from build123d import *

# Parameters (mm, degrees)
STOCK_TO_SIZE_DEPTH = 3.175
SKETCH2_R           = 2.286
MOUNTING_HOLE_DEPTH = 4.175


with BuildPart() as part:
    # Sketch1 → Stock to Size (new body)
    with BuildSketch(Plane(origin=(0, 0, 0), x_dir=(1, 0, 0), z_dir=(0, 1, 0))):
        with BuildLine():
            Line((-72.207668016, -239.550243772), (113.425121886, -239.550243772))
            ThreePointArc((113.425121886, -239.550243772), (117.915249947, -237.690371833), (119.775121886, -233.200243772))
            Line((119.775121886, -233.200243772), (119.775121886, 363.699756228))
            ThreePointArc((119.775121886, 363.699756228), (117.915249947, 368.189884288), (113.425121886, 370.049756228))
            Line((113.425121886, 370.049756228), (-154.880183722, 370.049756228))
            Line((-154.880183722, 370.049756228), (-180.160298169, 342.461352424))
            Line((-180.160298169, 342.461352424), (-78.461197248, -234.302909701))
            ThreePointArc((-78.461197248, -234.302909701), (-76.289369337, -238.064625986), (-72.207668016, -239.550243772))
        make_face()
    extrude(amount=STOCK_TO_SIZE_DEPTH)

    # Sketch2 → Mounting Hole (cut, through all)
    with BuildSketch(Plane(origin=(0, 3.175, 0), x_dir=(1, 0, 0), z_dir=(0, 1, 0))):
        with Locations((-43.86710003, -137.950243772)):
            Circle(SKETCH2_R)
    extrude(amount=-MOUNTING_HOLE_DEPTH, mode=Mode.SUBTRACT)


solid = part.part
The model under review builds one solid part; all positions refer to its coordinate system, in mm. Round coordinates to 2 decimals unless told otherwise and drop trailing zeros. Loops run counter-clockwise (first coordinate to the right, second up) from the corner with the lowest first, then second, coordinate; pieces in that order, holes last. Notation, with made-up numbers: (88.5, 27.25) -> (113.5, 27.25) arc R18 ccw to (113.5, 32.25) -> close; hole circle Ø8 at (40.5, 38.5). An arc over 180 degrees is marked (long way). Answer as CSV lines item,"result".
1) For P1, Ø1, axis at y = 2, z = -42.5, coming from the -X side; P2, Ø4, axis at x = -43.87, z = 137.95, coming from the -Y side, all flat-tipped, find the tip position at first contact; note any pin that passes through.
Geometry results:
P1,"stops at x = -127.36"
P2,"passes through"
2) Add section A-A on y = 1.75. Write out the cut boundary in (x, z).
Geometry results:
outline,"(-180.16, -342.46) -> (-154.88, -370.05) -> (113.43, -370.05) arc R6.35 ccw to (119.78, -363.7) -> (119.78, 233.2) arc R6.35 ccw to (113.43, 239.55) -> (-72.21, 239.55) arc R6.35 ccw to (-78.46, 234.3) -> close; hole circle Ø4.57 at (-43.87, 137.95)"
3) Add section C-C on x = -143. Write out the cut boundary in (y, z) (3 decimals).
Geometry results:
outline,"(0, -370.05) -> (3.175, -370.05) -> (3.175, -131.715) -> (0, -131.715) -> close"
4) Add section B-B on z = -139. Write out the cut boundary in (x, y) (3 decimals), plus the area to 3 significant figures.
Geometry results:
outline,"(-144.285, 0) -> (119.775, 0) -> (119.775, 3.175) -> (-144.285, 3.175) -> close"
area,"838 mm²"
5) To check wall thickness, follow line 1 along X through (y, z) = (2.35, 96.5); line 2 along X through (y, z) = (1.45, 23); line 3 along Z through (x, y) = (-75.5, 2.6). State the ranges of each line that lie inside material, in increasing order. Write a range as from..to.
Geometry results:
line 1,"x = -102.76..119.78"
line 2,"x = -115.72..119.78"
line 3,"z = -370.05..238.63"
